from build123d import *

# Parameters (mm, degrees)
F1_DEPTH      = 243
F3_DEPTH      = 20.001
F3_DEPTH_BACK = 20.001


# Not quite as in the source:
# - a pattern or mirror of a feature is missing from the dataset's text; its kind, count and spacing are read off the source's solid


with BuildPart() as f1:
    # F0 (on Top) → F1 (new body, symmetric)
    with BuildSketch(Plane.XY):
        with BuildLine():
            Line((17, 20), (-17, 20))
            ThreePointArc((-17, 20), (-19.1213203436, 19.1213203436), (-20, 17))
            Line((-20, 17), (-20, -17))
            ThreePointArc((-20, -17), (-19.1213203436, -19.1213203436), (-17, -20))
            Line((-17, -20), (17, -20))
            ThreePointArc((17, -20), (19.1213203436, -19.1213203436), (20, -17))
            Line((20, -17), (20, 17))
            ThreePointArc((20, 17), (19.1213203436, 19.1213203436), (17, 20))
        make_face()
        with BuildLine():
            ThreePointArc((-18, 17), (-17.7071067812, 17.7071067812), (-17, 18))
            Line((-17, 18), (17, 18))
            ThreePointArc((17, 18), (17.7071067812, 17.7071067812), (18, 17))
            Line((18, 17), (18, -17))
            ThreePointArc((18, -17), (17.7071067812, -17.7071067812), (17, -18))
            Line((17, -18), (-17, -18))
            ThreePointArc((-17, -18), (-17.7071067812, -17.7071067812), (-18, -17))
            Line((-18, -17), (-18, 17))
        make_face(mode=Mode.SUBTRACT)
    extrude(amount=F1_DEPTH, both=True)

    # F2 (on Front) → F3 (cut, two sides)
    with BuildSketch(Plane.XZ) as f3_sk:
        Polygon((20, 243), (-20, 243), (-20, 203), align=None)
    f3 = extrude(amount=-F3_DEPTH, mode=Mode.SUBTRACT) + extrude(f3_sk.sketch, amount=F3_DEPTH_BACK, mode=Mode.SUBTRACT)

    # F3_copies: F3 across plane
    add(f3.mirror(Plane(origin=(0, 0, 0), x_dir=(-1, 0, 0), z_dir=(0, 0, -1))), mode=Mode.SUBTRACT)


solid = f1.part
Can you work these out from the model? Positions are in its coordinate system, mm. A direction names the side the tool comes from. Round coordinates to 2 decimals unless told otherwise and drop trailing zeros. Order: outer loops, then holes, each group sorted by start corner. A loop starts at its lowest first (then second) coordinate and runs counter-clockwise, first axis right, second up. Notation, with made-up numbers: (-35, 12.5) - (15, 12.5) arc R32 ccw to (15, 43.5) - close; hole circle Ø10 at (41.25, -17.75). An arc over 180 degrees is marked (long way). Answer in a Markdown table with one row per item.
(1) Suppose I cut it at C-C, the plane y = 1.5. Please give me the cut outline in (x, z), plus the area to 3 significant figures.
From the geometry:
| item | result |
|---|---|
| outline | (-20, -203) - (-18, -205) - (-18, 205) - (-20, 203) - close; (18, -241) - (20, -243) - (20, 243) - (18, 241) - close |
| area | 1,780 mm2 |
(2) If we mould it in two halves opening along Y, with no side actions, what happens to faces 3 (the face through (0, -20, 3)), 4 (the face through (-20, 0, 3)), 5 (the face through (0, 18, 3))? For each: released by +Y, released by -Y, zero draft, split by the parting line, or undercut.
From the geometry:
| item | result |
|---|---|
| face 3 | released by -Y |
| face 4 | zero draft |
| face 5 | undercut |
(3) Suppose I cut it at A-A, the plane x = 0. Please give me the cut outline in (y, z), plus the area to 3 significant figures.
From the geometry:
| item | result |
|---|---|
| outline | (-20, -223) - (-18, -223) - (-18, 223) - (-20, 223) - close; (18, -223) - (20, -223) - (20, 223) - (18, 223) - close |
| area | 1,780 mm2 |
(4) Which directions (+Z, -Z, +X, -X, +Y, -Y) give clear straight access to the entire face, cutting with the end or side of a thin tool? Please do faces 1 (the face through (0, -19, -223)), 2 (the face through (0, -18, 3)).
From the geometry:
| item | result |
|---|---|
| face 1 | -Z, -X, +Y, -Y |
| face 2 | +Z, -Z |
(5) For P1, Ø10, axis at x = 1, y = 12, coming from the +Z side, with a flat end and sliding along its axis, tell me the tip position at first contact or that it passes through.
From the geometry:
| item | result |
|---|---|
| P1 | passes through |
(6) Suppose I cut it at B-B, the plane z = -68.5. Please give me the cut outline in (x, y), plus the area to 3 significant figures.
From the geometry:
| item | result |
|---|---|
| outline | (-20, -17) arc R3 ccw to (-17, -20) - (17, -20) arc R3 ccw to (20, -17) - (20, 17) arc R3 ccw to (17, 20) - (-17, 20) arc R3 ccw to (-20, 17) - close; hole (-18, -17) arc R1 ccw to (-17, -18) - (17, -18) arc R1 ccw to (18, -17) - (18, 17) arc R1 ccw to (17, 18) - (-17, 18) arc R1 ccw to (-18, 17) - close |
| area | 297 mm2 |
(7) Please list where these lines run through material, in increasing order: L1, parallel to X at y = 7, z = -137.5; L2, parallel to X at y = 18.5, z = -37.5. Write a range as from..to.
From the geometry:
| item | result |
|---|---|
| L1 | x = -20..-18, 18..20 |
| L2 | x = -19.6..19.6 |
